The listing builds one solid part. Answer for the finished solid, in the listing's coordinates (mm). A direction names the side the tool comes from. Give positions to 0.01 mm unless a question says otherwise; leave off trailing zeros. Write each loop counter-clockwise with the first axis right and the second up, starting at its lowest first coordinate (ties: lowest second). Pieces come first, ordered by that corner, then holes. Notation, with made-up numbers: M -33,54 L 25,54 A15 cw 25,68 Z; hole C 16,16 d11. An arc over 180 degrees is marked long. Answer as a JSON object with one key per item and string values.
```python
from build123d import *

# Parameters (mm, degrees)
F1_DEPTH = 25
F3_D     = 10.8
F3_DEPTH = 21
F3_TIP   = 3.2446473427
F5_D     = 8.8
F5_DEPTH = 21
F5_TIP   = 2.6437867237
F6_R     = 0.5


with BuildPart() as f1:
    # F0 (on Front) → F1 (new body)
    with BuildSketch(Plane.XZ):
        Polygon((0, -20), (0, 0), (-30, 0), (-30, 50), (30, 50), (30, 70), (-50, 70), (-50, -20), align=None)
    extrude(amount=F1_DEPTH)

    # F3 (one way)
    with BuildSketch(Plane(origin=(0, 0, 50), x_dir=(1, 0, 0), z_dir=(0, 0, -1))):
        with Locations((-12, 12.5)):
            Circle(F3_D / 2)
    extrude(amount=-F3_DEPTH, mode=Mode.SUBTRACT)
    with Locations(Plane(origin=(0, 0, 50), x_dir=(1, 0, 0), z_dir=(0, 0, -1))):
        with Locations((-12, 12.5)):
            with Locations((0, 0, -(F3_DEPTH + F3_TIP / 2))):  # 118° drill point
                Cone(0, F3_D / 2, F3_TIP, mode=Mode.SUBTRACT)

    # F5
    with Locations(Plane.YZ.offset(30)):
        with Locations((-12.5, 60)):
            Hole(F5_D / 2, depth=F5_DEPTH)
            with Locations((0, 0, -(F5_DEPTH + F5_TIP / 2))):  # 118° drill point
                Cone(0, F5_D / 2, F5_TIP, mode=Mode.SUBTRACT)

    # F6
    f6_edges = [f1.edges().sort_by_distance(p)[0] for p in [
        (0, -25, -10),
        (-15, -25, 0),
        (-30, -25, 25),
        (0, -25, 50),
        (30, -25, 60),
        (-10, -25, 70),
        (-50, -25, 25),
        (-25, -25, -20),
        (0, 0, -10),
        (-15, 0, 0),
        (-30, 0, 25),
        (0, 0, 50),
        (30, 0, 60),
        (-10, 0, 70),
        (-50, 0, 25),
        (-25, 0, -20),
        (30, -12.5, 70),
        (30, -12.5, 50),
        (0, -12.5, -20),
        (0, -12.5, 0),
        (-50, -12.5, -20),
        (-50, -12.5, 70),
        (-17.4, -12.5, 50),
        (30, -16.9, 60),
        (-17.4, -12.5, 70),
    ]]
    fillet(f6_edges, radius=F6_R)


solid = f1.part
```
1. A cutting plane is placed at A-A, the plane x = -12. Give the vertices of the cut face in (y, z), plus the area to 3 significant figures.
Verdict:
{"outline": "M -25,-19.5 A0.5 ccw -24.5,-20 L -0.5,-20 A0.5 ccw 0,-19.5 L 0,-0.5 A0.5 ccw -0.5,0 L -24.5,0 A0.5 ccw -25,-0.5 Z; M -25,50.5 A0.5 ccw -24.5,50 L -18.4,50 A0.5 ccw -17.9,50.5 L -17.9,69.5 A0.5 ccw -18.4,70 L -24.5,70 A0.5 ccw -25,69.5 Z; M -7.1,50.5 A0.5 ccw -6.6,50 L -0.5,50 A0.5 ccw 0,50.5 L 0,69.5 A0.5 ccw -0.5,70 L -6.6,70 A0.5 ccw -7.1,69.5 Z", "area": "783 mm2"}
2. Flat-ended cylindrical pins translate along their axes: pin 1 (7 mm diameter, centred on y = -12.5, z = 60, fed in from +X); pin 2 (8 mm diameter, centred on x = 6.5, y = -22, fed in from -Z). Find the tip coordinate at first contact, or state that the pin passes through.
Verdict:
{"pin 1": "stops at x = 8.46", "pin 2": "stops at z = 50"}
3. A cutting plane is placed at D-D, the plane z = 27.5. Give the vertices of the cut face in (x, y).
Verdict:
{"outline": "M -50,-24.5 A0.5 ccw -49.5,-25 L -30.5,-25 A0.5 ccw -30,-24.5 L -30,-0.5 A0.5 ccw -30.5,0 L -49.5,0 A0.5 ccw -50,-0.5 Z"}
4. A cutting plane is placed at C-C, the plane z = -6. Give the vertices of the cut face in (x, y), plus the area to 3 significant figures.
Verdict:
{"outline": "M -50,-24.5 A0.5 ccw -49.5,-25 L -0.5,-25 A0.5 ccw 0,-24.5 L 0,-0.5 A0.5 ccw -0.5,0 L -49.5,0 A0.5 ccw -50,-0.5 Z", "area": "1,250 mm2"}
5. A cutting plane is placed at B-B, the plane y = -5. Give the vertices of the cut face in (x, z).
Verdict:
{"outline": "M -50,-19.5 A0.5 ccw -49.5,-20 L -0.5,-20 A0.5 ccw 0,-19.5 L 0,-0.5 A0.5 ccw -0.5,0 L -30,0 L -30,50 L 29.5,50 A0.5 ccw 30,50.5 L 30,69.5 A0.5 ccw 29.5,70 L -49.5,70 A0.5 ccw -50,69.5 Z"}
6. The mould has two halves that part along Z. Classify faces 5 (the flat face through (-15, -12, 0)), 6 (the flat face through (-37, 0, 36)), 7 (the flat face through (-9, -7, 70)): released by +Z, released by -Z, zero draft, split by the parting line, or undercut.
Verdict:
{"face 5": "undercut", "face 6": "zero draft", "face 7": "released by +Z"}
7. Consider line 1 along Z through (x, y) = (-1.5, -8.5); line 2 along Y through (x, z) = (-12, 63); line 3 along Z through (x, y) = (22.5, -12.5). Determine where each line is inside the solid, lowest interval first.
Verdict:
{"line 1": "z = -20 to 0, 50 to 70", "line 2": "y = -25 to -17.9, -7.1 to 0", "line 3": "z = 50 to 55.6, 64.4 to 70"}
8. For faces 1 (the cylindrical face through (-9.51, -7.71, 59.87)), 2 (the cylindrical face through (19.106, -11.546, 55.705)), 3 (the flat face through (0, -12, -10)), 4 (the flat face through (-1, -12, 50)), determine the directions among +Z, -Z, +X, -X, +Y, -Y from which every point of the face is accessible in a straight line to the end or side of a thin tool.
Verdict:
{"face 1": "+Z", "face 2": "+X", "face 3": "-Z, +X, +Y, -Y", "face 4": "+X, +Y, -Y"}
